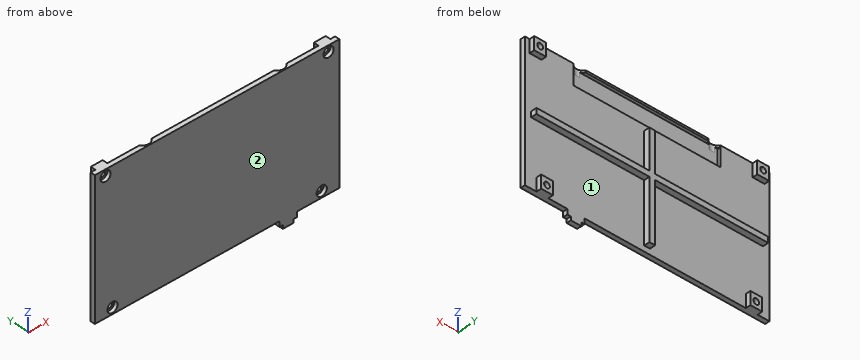
```python
from build123d import *

# Parameters (mm, degrees)
SKETCH1_W            = 136.0932
SKETCH1_H            = 77.343
BOSS_EXTRUDE1_DEPTH  = 2.54
SKETCH2_R            = 3.8735
CUT_EXTRUDE1_DEPTH   = 3.81
SKETCH3_W            = 81.691378436
SKETCH3_H            = 10.2362
CUT_EXTRUDE2_DEPTH   = 1.651
SKETCH4_W            = 6.604
SKETCH4_H            = 7.366
BOSS_EXTRUDE4_DEPTH  = 2.794
SKETCH5_R            = 2.8575
CUT_EXTRUDE3_DEPTH   = 2.032
M3_CLEARANCE_HOLE1_D = 3.2
SKETCH9_W            = 9.652
SKETCH9_H            = 2.54
BOSS_EXTRUDE5_DEPTH  = 2.921
SKETCH10_W           = 5.842
SKETCH10_H           = 2.54
BOSS_EXTRUDE6_DEPTH  = 2.032
BOSS_EXTRUDE7_DEPTH  = 3.175


with BuildPart() as part:
    # Sketch1 → Boss-Extrude1 (new body)
    with BuildSketch(Plane(origin=(0, 0, 0), x_dir=(1, 0, 0), z_dir=(0, 1, 0))):
        with Locations((68.0466, 38.6715)):
            Rectangle(SKETCH1_W, SKETCH1_H)
    extrude(amount=BOSS_EXTRUDE1_DEPTH)

    # Sketch2 → Cut-Extrude1 (cut)
    with BuildSketch(Plane.XY):
        with Locations((105.5477, 4.4939)):
            Circle(SKETCH2_R)
        with Locations((30.5455, 4.4939)):
            Circle(SKETCH2_R)
    extrude(amount=-CUT_EXTRUDE1_DEPTH, mode=Mode.SUBTRACT)

    # Sketch3 → Cut-Extrude2 (cut)
    with BuildSketch(Plane(origin=(0, 2.54, 0), x_dir=(1, 0, 0), z_dir=(0, 1, 0))):
        with Locations((68.0466, 6.3119)):
            Rectangle(SKETCH3_W, SKETCH3_H)
    extrude(amount=-CUT_EXTRUDE2_DEPTH, mode=Mode.SUBTRACT)

    # Sketch4 → Boss-Extrude4 (add)
    with BuildSketch(Plane(origin=(0, 2.54, 0), x_dir=(1, 0, 0), z_dir=(0, 1, 0))):
        with Locations((130.1242, 3.683)):
            Rectangle(SKETCH4_W, SKETCH4_H)
        with Locations((5.969, 3.683)):
            Rectangle(SKETCH4_W, SKETCH4_H)
        with Locations((126.3142, 73.66)):
            Rectangle(SKETCH4_W, SKETCH4_H)
        with Locations((9.779, 73.66)):
            Rectangle(SKETCH4_W, SKETCH4_H)
    extrude(amount=BOSS_EXTRUDE4_DEPTH)

    # Sketch5 → Cut-Extrude3 (cut)
    with BuildSketch(Plane(origin=(0, 0, 0), x_dir=(-1, 0, 0), z_dir=(0, -1, 0))):
        with Locations((-126.3142, 73.787)):
            Circle(SKETCH5_R)
        with Locations((-9.8044, 73.787)):
            Circle(SKETCH5_R)
        with Locations((-5.969, 3.556)):
            Circle(SKETCH5_R)
        with Locations((-130.1242, 3.556)):
            Circle(SKETCH5_R)
    extrude(amount=-CUT_EXTRUDE3_DEPTH, mode=Mode.SUBTRACT)

    # M3 Clearance Hole1 (through all)
    with Locations(Plane(origin=(0, 2.032, 0), x_dir=(-1, 0, 0), z_dir=(0, -1, 0))):
        with Locations((-5.969, 3.556), (-130.1242, 3.556), (-126.3142, 73.787), (-9.8044, 73.787)):
            Hole(M3_CLEARANCE_HOLE1_D / 2)

    # Sketch9 → Boss-Extrude5 (add)
    with BuildSketch(Plane(origin=(0, 0, -77.343), x_dir=(-1, 0, 0), z_dir=(0, 0, -1))):
        with Locations((-107.5944, 1.27)):
            Rectangle(SKETCH9_W, SKETCH9_H)
    extrude(amount=BOSS_EXTRUDE5_DEPTH)

    # Sketch10 → Boss-Extrude6 (add)
    with BuildSketch(Plane(origin=(0, 0, -80.264), x_dir=(-1, 0, 0), z_dir=(0, 0, -1))):
        with Locations((-107.5944, 1.27)):
            Rectangle(SKETCH10_W, SKETCH10_H)
    extrude(amount=BOSS_EXTRUDE6_DEPTH)

    # Sketch11 → Boss-Extrude7 (add)
    with BuildSketch(Plane(origin=(0, 2.54, 0), x_dir=(1, 0, 0), z_dir=(0, 1, 0))):
        Polygon((132.5372, 37.084), (69.6341, 37.084), (69.6341, 14.605), (66.4591, 14.605), (66.4591, 37.084), (3.556, 37.084), (3.556, 40.259), (66.4591, 40.259), (66.4591, 74.168), (69.6341, 74.168), (69.6341, 40.259), (132.5372, 40.259), align=None)
    extrude(amount=BOSS_EXTRUDE7_DEPTH)


solid = part.part
```
Check sheet for the modelled part. Datum: model origin and axes. Units: mm. Face numbers are marked on the shaded views. A direction names the side the tool comes from. Round coordinates to 2 decimals unless told otherwise and drop trailing zeros. Loops run counter-clockwise (first coordinate to the right, second up) from the corner with the lowest first, then second, coordinate; pieces in that order, holes last. Notation, with made-up numbers: (27.25, -3.75) - (72.25, -3.75) arc R17 cw to (72.25, 9.25) - close; hole circle Ø11 at (-30, -5.75). An arc over 180 degrees is marked (long way). Answer as a JSON object with one key per item and string values. Group by question number.
Q1. Set-up check for the marked faces 1 and 2: record each of +Z, -Z, +X, -X, +Y, -Y from which the full face is reachable in a straight line by a thin tool's end or side.
Q2. Scan lines: line 1 along X through (y, z) = (3.5, -71); line 2 along Z through (x, y) = (126, 2.85); line 3 along Z through (x, y) = (123.5, 5.1). Record each from-to range of solid material in increasing order. Write a range as [from, to].
Q3. Sectioned sample at A-A, the plane x = 88.5. Enter the section's corners in (y, z) (3 decimals), plus the area to 3 significant figures.
Q4. Sectioned sample at C-C, the plane z = -54.5. Enter the section's corners in (x, y) (3 decimals).
Q5. Sectioned sample at D-D, the plane x = 24.5. Enter the section's corners in (y, z) (3 decimals), plus the area to 3 significant figures.
Q6. Gauge pin test, flat ends, axial feed: P1, Ø2.5, axis at y = 5, z = -39.5, coming from the -X side; P2, Ø3.5, axis at x = 5.969, z = -3.556, coming from the +Y side; P3, Ø1.8, axis at x = 28, y = 1.5, coming from the -Z side. Record the tip position at first contact, or that the pin passes through.
Q7. Sectioned sample at B-B, the plane y = 4.2. Count the separate pieces of the cut face and the enclosed holes in it, plus the area to 3 significant figures.
Solution:
{
 "1": {"face 1": "+Y", "face 2": "+Z, -Z, +X, -X, -Y"},
 "2": {"line 1": "x = [6.48, 13.08], [66.46, 69.63], [123.01, 129.62]", "line 2": "z = [-77.34, -75.36], [-72.22, -69.98], [-40.26, -37.08]", "line 3": "z = [-77.34, -69.98], [-40.26, -37.08]"},
 "3": {"outline": "(0, -77.343) - (2.54, -77.343) - (2.54, -40.259) - (5.715, -40.259) - (5.715, -37.084) - (2.54, -37.084) - (2.54, -11.43) - (0.889, -11.43) - (0.889, -1.194) - (2.54, -1.194) - (2.54, 0) - (0, 0) - close", "area": "190 mm²"},
 "4": {"outline": "(0, 0) - (136.093, 0) - (136.093, 2.54) - (69.634, 2.54) - (69.634, 5.715) - (66.459, 5.715) - (66.459, 2.54) - (0, 2.54) - close"},
 "5": {"outline": "(0, -77.343) - (2.54, -77.343) - (2.54, -40.259) - (5.715, -40.259) - (5.715, -37.084) - (2.54, -37.084) - (2.54, 0) - (0, 0) - close", "area": "207 mm²"},
 "6": {"P1": "stops at x = 3.56", "P2": "stops at y = 5.33", "P3": "stops at z = -77.34"},
 "7": {"separate pieces": "5", "enclosed holes": "4", "area": "751 mm²"}
}
